Model file for the job. Use its own axes, mm. Round coordinates to 2 decimals unless told otherwise and drop trailing zeros. Order: outer loops, then holes, each group sorted by start corner. A loop starts at its lowest first (then second) coordinate and runs counter-clockwise, first axis right, second up. Notation, with made-up numbers: (41, -32.75) - (64, -32.75) arc R19 cw to (64, -4.75) - close; hole circle Ø8 at (35.5, 35.25). An arc over 180 degrees is marked (long way). Put each result on its own line as item: value. Start each with the question number.
Item 1: Saw through at D-D on x = -14.5. List the corners of the cut face in (y, z).
Item 2: Pin check, flat tips, straight feed: pin 1 Ø1.5 at (y, z) = (10, -34) entering from -X; pin 2 Ø1 at (y, z) = (16, -15.5) entering from -X; pin 3 Ø2 at (x, y) = (19.5, 3.5) entering from -Z. Stop position of each tip, or through.
Item 3: Saw through at A-A on z = 7.5. List the corners of the cut face in (x, y).
Item 4: Saw through at B-B on x = 0. List the corners of the cut face in (y, z).
Item 5: Probe probe 1 along X at (y, z) = (16, 7.5); probe 2 along X at (y, z) = (1.5, -1); probe 3 along X at (y, z) = (5.75, -23). List the from-to ranges inside material, lowest first.
Item 6: Saw through at C-C on y = 2.25. List the corners of the cut face in (x, z), plus the area to 3 significant figures.
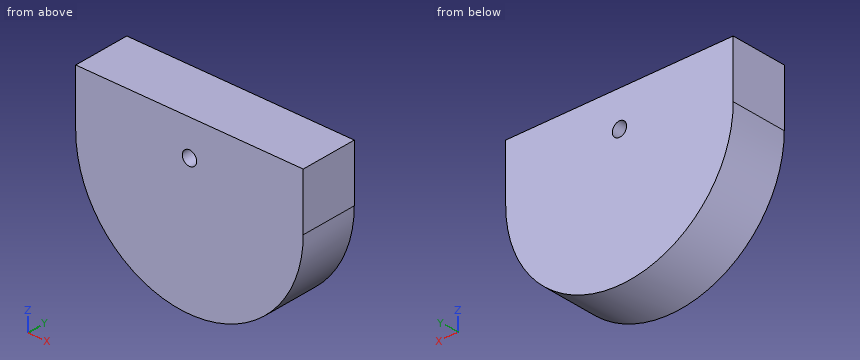
```python
from build123d import *

# Parameters (mm, degrees)
BOSS_EXTRUDE1_DEPTH = 20
SKETCH3_W           = 80
SKETCH3_H           = 15
BOSS_EXTRUDE3_DEPTH = 20
SKETCH4_R           = 1.75
CUT_EXTRUDE1_DEPTH  = 20
SKETCH6_W           = 80
SKETCH6_H           = 5
BOSS_EXTRUDE4_DEPTH = 20
SKETCH7_R           = 2.518213347
CUT_EXTRUDE3_DEPTH  = 20


with BuildPart() as part:
    # Sketch1 → Boss-Extrude1 (new body)
    with BuildSketch(Plane(origin=(0, 0, 0), x_dir=(1, 0, 0), z_dir=(0, 1, 0))):
        with BuildLine():
            Line((-40, 0), (40, 0))
            ThreePointArc((40, 0), (0, 40), (-40, 0))
        make_face()
    extrude(amount=BOSS_EXTRUDE1_DEPTH)

    # Sketch3 → Boss-Extrude3 (add)
    with BuildSketch(Plane(origin=(0, 20, 0), x_dir=(1, 0, 0), z_dir=(0, 1, 0))):
        with Locations((0, -7.5)):
            Rectangle(SKETCH3_W, SKETCH3_H)
    extrude(amount=-BOSS_EXTRUDE3_DEPTH)

    # Sketch4 → Cut-Extrude1 (cut)
    with BuildSketch(Plane(origin=(0, 0, 0), x_dir=(-1, 0, 0), z_dir=(0, -1, 0))):
        with Locations(Location((0, -7.5, 0), (0, 0, 90))):
            Circle(SKETCH4_R)
    extrude(amount=-CUT_EXTRUDE1_DEPTH, mode=Mode.SUBTRACT)

    # Sketch6 → Boss-Extrude4 (add)
    with BuildSketch(Plane(origin=(0, 0, 0), x_dir=(-1, 0, 0), z_dir=(0, -1, 0))):
        with Locations((0, -17.5)):
            Rectangle(SKETCH6_W, SKETCH6_H)
    extrude(amount=-BOSS_EXTRUDE4_DEPTH)

    # Sketch7 → Cut-Extrude3 (cut)
    with BuildSketch(Plane(origin=(0, 20, 0), x_dir=(1, 0, 0), z_dir=(0, 1, 0))):
        with Locations(Location((0, -7.5, 0), (0, 0, 270))):
            Circle(SKETCH7_R)
    extrude(amount=-CUT_EXTRUDE3_DEPTH, mode=Mode.SUBTRACT)


solid = part.part
```
Results found:
1. outline: (0, -37.28) - (20, -37.28) - (20, 20) - (0, 20) - close
2. pin 1: stops at x = -22.24
2. pin 2: stops at x = -37.08
2. pin 3: stops at z = -35.46
3. outline: (-40, 0) - (-2.52, 0) - (-2.52, 20) - (-40, 20) - close; (2.52, 0) - (40, 0) - (40, 20) - (2.52, 20) - close
4. outline: (0, -40) - (20, -40) - (20, 4.98) - (0, 4.98) - close; (0, 10.02) - (20, 10.02) - (20, 20) - (0, 20) - close
5. probe 1: x = -40 to -2.52, 2.52 to 40
5. probe 2: x = -39.99 to 39.99
5. probe 3: x = -32.73 to 32.73
6. outline: (-40, 0) arc R40 ccw to (40, 0) - (40, 20) - (-40, 20) - close; hole circle Ø5.04 at (0, 7.5)
6. area: 4,090 mm²
